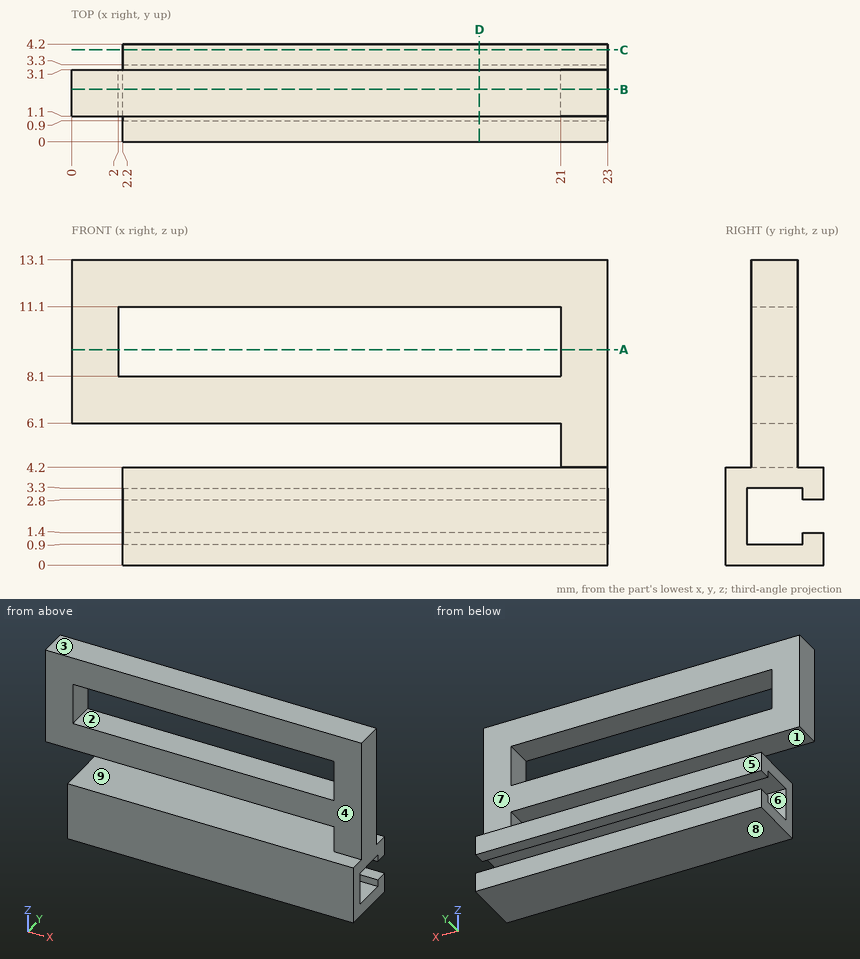
The figure shows three views and two pictorial views of one solid part (mm, origin at its lowest corner). Answer the questions. A direction names the side the tool comes from. Coordinates: 2 decimals unless noted, no trailing zeros. Loops run counter-clockwise (first coordinate to the right, second up) from the corner with the lowest first, then second, coordinate; pieces in that order, holes last.
1) Find section C-C on y = 3.95. Write down the section's boundary in (x, z).
2) A tool of negligible diameter and unlimited length cuts with its end or side. For the marked faces 1, 2, 3, 4 and 5, from which of +Z, -Z, +X, -X, +Y, -Y can it reach the whole face along a straight path? Write none if from no direction.
3) Find section A-A on z = 9.25. Write down the section's boundary in (x, y).
4) Find section D-D on x = 17.5. Write down the section's boundary in (y, z), then the cut area to 3 significant figures.
5) Find section B-B on y = 2.25. Write down the section's boundary in (x, z), then the cut area to 3 significant figures.
6) Flat-ended cylindrical pins translate along their axes: pin 1 Ø6 at (x, z) = (17, 11.5) entering from +Y; pin 2 Ø1 at (x, z) = (13.5, 7.5) entering from -Y; pin 3 Ø2 at (y, z) = (2, 5) entering from -X. Find the tip coordinate at first contact, or state that the pin passes through.
7) Find the intervals of material crossed by L1, parallel to Z at x = 5.75, y = 2.1; L2, parallel to X at y = 1.8, z = 10.5; L3, parallel to Z at x = 21.25, y = 3.45, in increasing order.
8) Determine the mould class of the marked faces 6, 7, 8 and 9 for opening direction Z: pulls with the +Z half, pulls with the -Z half, needs draft (parallel to the pull), parting line crosses it, or undercut.
Values:
1. outline: (2.2, 0) - (23, 0) - (23, 1.4) - (2.2, 1.4) - close; (2.2, 2.8) - (23, 2.8) - (23, 4.2) - (2.2, 4.2) - close
2. face 1: -X, +Y, -Y
2. face 2: +Y, -Y
2. face 3: +Z, +X, -X, +Y, -Y
2. face 4: +Z, +X, -X, -Y
2. face 5: +Z, -Z, +X, -X, +Y
3. outline: (0, 1.1) - (2, 1.1) - (2, 3.1) - (0, 3.1) - close; (21, 1.1) - (23, 1.1) - (23, 3.1) - (21, 3.1) - close
4. outline: (0, 0) - (4.2, 0) - (4.2, 1.4) - (3.3, 1.4) - (3.3, 0.9) - (0.9, 0.9) - (0.9, 3.3) - (3.3, 3.3) - (3.3, 2.8) - (4.2, 2.8) - (4.2, 4.2) - (0, 4.2) - close; (1.1, 6.1) - (3.1, 6.1) - (3.1, 8.1) - (1.1, 8.1) - close; (1.1, 11.1) - (3.1, 11.1) - (3.1, 13.1) - (1.1, 13.1) - close
4. area: 18.6 mm2
5. outline: (0, 6.1) - (21, 6.1) - (21, 4.2) - (2.2, 4.2) - (2.2, 3.3) - (23, 3.3) - (23, 13.1) - (0, 13.1) - close; (2.2, 0) - (23, 0) - (23, 0.9) - (2.2, 0.9) - close; hole (2, 8.1) - (21, 8.1) - (21, 11.1) - (2, 11.1) - close
5. area: 145 mm2
6. pin 1: stops at y = 3.1
6. pin 2: stops at y = 1.1
6. pin 3: stops at x = 2.2
7. L1: z = 0 to 0.9, 3.3 to 4.2, 6.1 to 8.1, 11.1 to 13.1
7. L2: x = 0 to 2, 21 to 23
7. L3: z = 0 to 1.4, 2.8 to 4.2
8. face 6: undercut
8. face 7: needs draft
8. face 8: pulls with the -Z half
8. face 9: undercut
